Autodesk Inventor part; units mm, degrees
ref_plane "YZ Plane" through (0, 0, 0) normal (1, 0, 0) x (0, 1, 0)
ref_plane "XZ Plane" through (0, 0, 0) normal (0, 1, 0) x (-1, 0, 0)
ref_plane "XY Plane" through (0, 0, 0) normal (0, 0, 1) x (1, 0, 0)
sketch "Sketch2" plane through (0, 0, 0) normal (0, 0, 1) x (1, 0, 0)
  line L0 (-5.0655, 3.6572) -> (12.9345, 3.6572)
  line L1 (12.9345, 3.6572) -> (12.9345, -8.3428)
  line L2 (12.9345, -8.3428) -> (-5.0655, -8.3428)
  line L3 (-5.0655, -8.3428) -> (-5.0655, 3.6572)
  line L4 (8.9345, 3.6572) -> (7.7095, 0.3786)
  line L5 (7.7095, 0.3786) -> (-1.0655, 3.6572)
  line L6 (-1.0655, 3.6572) -> (-1.0655, 11.6572)
  line L7 (-1.0655, 11.6572) -> (8.9345, 11.6572)
  line L8 (8.9345, 11.6572) -> (8.9345, 3.6572)
  point P0 (0, 0)
  dimension "d0" = 18
  dimension "d1" = 12
  dimension "d2" = 3.5
  dimension "d3" = 4
  dimension "d4" = 4
  dimension "d5" = 110.487
  dimension "d6" = 8
extrude "Extrusion1" add sketch "Sketch2" along normal blind 9.5 contours L6 L7 L8 L0 | L0 L4 L5
sketch "Sketch3" plane through (0, 0, 9.5) normal (0, 0, 1) x (1, 0, 0)
  line L0 (-1.0655, 3.6572) -> (7.7095, 0.3786)
  line L1 (7.7095, 0.3786) -> (8.9345, 3.6572)
  line L2 (8.9345, 3.6572) -> (8.9345, 11.6572)
  line L3 (8.9345, 11.6572) -> (-1.0655, 11.6572)
  line L4 (-1.0655, 11.6572) -> (-1.0655, 3.6572)
  line L5 (-0.5655, 15.4431) -> (8.4345, 15.4431)
  line L6 (8.4345, 15.4431) -> (8.4345, -6.1671)
  line L7 (8.4345, -6.1671) -> (-0.5655, -6.1671)
  line L8 (-0.5655, -6.1671) -> (-0.5655, 15.4431)
  point P0 (0, 0)
  dimension "d9" = 0.5
  dimension "d10" = 0.5
extrude "Extrusion2" cut sketch "Sketch3" against normal blind 10 contours L8 L3 L6 L1 L0 | L0 L1 L6 L7 L8 | L8 L5 L6 L3 keep common part
sketch "Sketch4" plane through (-0.5655, 11.6572, 9.5) normal (0, 1, 0) x (1, 0, 0)
  line L0 (0, 0) -> (0, 9.5)
  line L1 (9, 0) -> (0, 0)
  line L2 (9, 9.5) -> (9, 0)
  line L3 (9, 9.5) -> (0, 9.5)
  point P0 (0.5655, 9.5)
  point P1 (4.5, 4.5)
  dimension "d13" = 4.5
  dimension "d14" = 4.5
  dimension "d15" = 9
  dimension "d16" = 9.5
hole "Hole1" at (3.9345, 11.6572, 5) direction (0, -1, 0) diameter 2.5 depth 7 tip angle 118
properties part number "3DP_PLA_Measurement_Rail_Rammer"
Can you work these out from the model? Positions are in its coordinate system, mm. Coordinates: 2 decimals unless noted, no trailing zeros. Loops run counter-clockwise (first coordinate to the right, second up) from the corner with the lowest first, then second, coordinate; pieces in that order, holes last. Notation, with made-up numbers: M -14,70.25 L 9,70.25 A13 cw 9,74.25 Z; hole C 59,23 d5. An arc over 180 degrees is marked long. Answer as CSV lines item,"result". Start each with the question number.
1. Suppose I cut it at D-D, the plane y = 3. List the corners of the cut face in (x, z) for me.
2. Suppose I cut it at B-B, the plane y = 4.5. List the corners of the cut face in (x, z) for me, plus the area to 3 significant figures.
3. For pin 1 Ø5 at (x, z) = (5, 3.5) entering from -Y, with a flat end and sliding along its axis, tell me the tip position at first contact or that it passes through.
4. If I drill on probe 1 along X at (y, z) = (7.5, 5); probe 2 along X at (y, z) = (5.5, 5.5); probe 3 along Z at (x, y) = (3.25, 8.25), over which ranges is the centre line in solid material (lowest first)? Write a range as [from, to].
5. Suppose I cut it at A-A, the plane z = 8.5. List the corners of the cut face in (x, y) for me, plus the area to 3 significant figures.
6. Thinking about a two-plate mould opening in X: for faces 1 (the face through (8.077, 1.362, 4.684)), 2 (the face through (2.7, 8.1, 4.8)), 3 (the face through (3.9, 11.657, 3.6)), which applies, +X half, -X half, draft (parallel to the pull), parting line (faces both ways), or undercut?
7. Suppose I cut it at C-C, the plane x = 0.75. List the corners of the cut face in (y, z) for me.
Output:
1,outline,"M 0.69,0 L 8.43,0 L 8.43,9.5 L 0.69,9.5 Z"
2,outline,"M -0.57,0 L 8.43,0 L 8.43,9.5 L -0.57,9.5 Z; hole C 3.93,5 d1.98"
2,area,"82.4 mm^2"
3,pin 1,"stops at y = 0.46"
4,probe 1,"x = [-0.57, 2.68], [5.18, 8.43]"
4,probe 2,"x = [-0.57, 2.79], [5.08, 8.43]"
4,probe 3,"z = [0, 3.95], [6.05, 9.5]"
5,outline,"M -0.57,3.47 L 7.71,0.38 L 8.43,2.32 L 8.43,11.66 L -0.57,11.66 Z"
5,area,"88.0 mm^2"
6,face 1,"+X half"
6,face 2,"undercut"
6,face 3,"draft"
7,outline,"M 2.98,0 L 11.66,0 L 11.66,9.5 L 2.98,9.5 Z"
